Answer from the drawing. Dimensions are ordinates in mm from the lowest x, y and z of the part. A direction names the side the tool comes from. Coordinates: 2 decimals unless noted, no trailing zeros. Order: outer loops, then holes, each group sorted by start corner. A loop starts at its lowest first (then second) coordinate and runs counter-clockwise, first axis right, second up. Notation, with made-up numbers: (27, 77.25) -> (75, 77.25) arc R22 cw to (75, 105.25) -> close; hole circle Ø4 at (69, 24). An arc over 180 degrees is marked (long way). Answer in a Markdown table with one row per item.
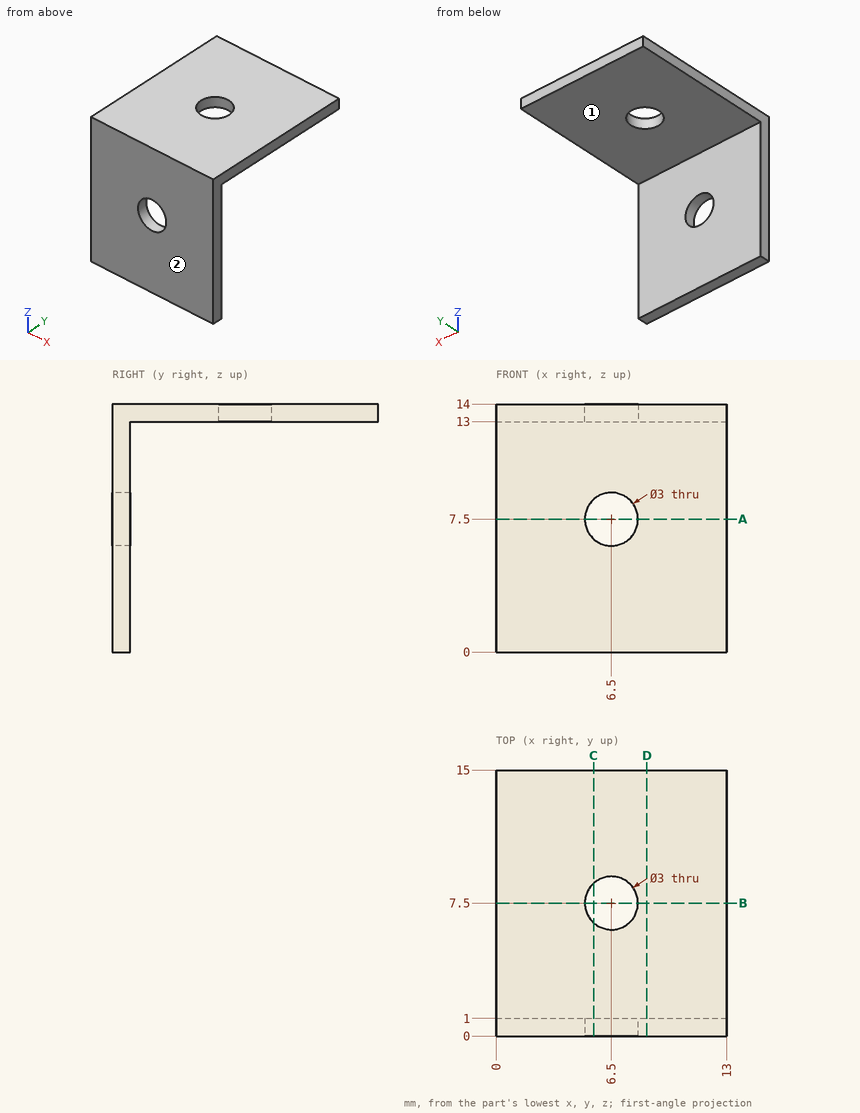
(1) Flat-ended cylindrical pins translate along their axes: pin 1 (1 mm diameter, centred on x = 3.5, z = 9.5, fed in from -Y); pin 2 (2 mm diameter, centred on x = 3, y = 12, fed in from -Z). Find the tip coordinate at first contact, or state that the pin passes through.
Check values:
| item | result |
|---|---|
| pin 1 | y = 0 |
| pin 2 | z = 13 |
(2) Find the intervals of material crossed by line 1 along Y through (x, z) = (6.5, 13.5); line 2 along Y through (x, z) = (12.5, 8.5); line 3 along Z through (x, y) = (5.75, 10.75), in increasing order. Write a range as from..to.
Check values:
| item | result |
|---|---|
| line 1 | 0..6, 9..15 |
| line 2 | 0..1 |
| line 3 | 13..14 |
(3) A cutting plane is placed at D-D, the plane x = 8.5. Determine the outline of the cut face in (y, z).
Check values:
| item | result |
|---|---|
| outline | (0, 0) -> (1, 0) -> (1, 13) -> (15, 13) -> (15, 14) -> (0, 14) -> close |
(4) A cutting plane is placed at B-B, the plane y = 7.5. Determine the outline of the cut face in (x, z), then the cut area to 3 significant figures.
Check values:
| item | result |
|---|---|
| outline | (0, 13) -> (5, 13) -> (5, 14) -> (0, 14) -> close; (8, 13) -> (13, 13) -> (13, 14) -> (8, 14) -> close |
| area | 10.0 mm² |
(5) Which of the six approach directions +Z, -Z, +X, -X, +Y, -Y give full straight-line access (tool end or side, diameter ignored) to the marked faces 1 and 2?
Check values:
| item | result |
|---|---|
| face 1 | -Z, +X, -X, +Y |
| face 2 | +Z, -Z, +X, -X, -Y |
(6) A cutting plane is placed at C-C, the plane x = 5.5. Determine the outline of the cut face in (y, z).
Check values:
| item | result |
|---|---|
| outline | (0, 0) -> (1, 0) -> (1, 6.38) -> (0, 6.38) -> close; (0, 8.62) -> (1, 8.62) -> (1, 13) -> (6.38, 13) -> (6.38, 14) -> (0, 14) -> close; (8.62, 13) -> (15, 13) -> (15, 14) -> (8.62, 14) -> close |
(7) A cutting plane is placed at A-A, the plane z = 7.5. Determine the outline of the cut face in (x, y), then the cut area to 3 significant figures.
Check values:
| item | result |
|---|---|
| outline | (0, 0) -> (5, 0) -> (5, 1) -> (0, 1) -> close; (8, 0) -> (13, 0) -> (13, 1) -> (8, 1) -> close |
| area | 10.0 mm² |
